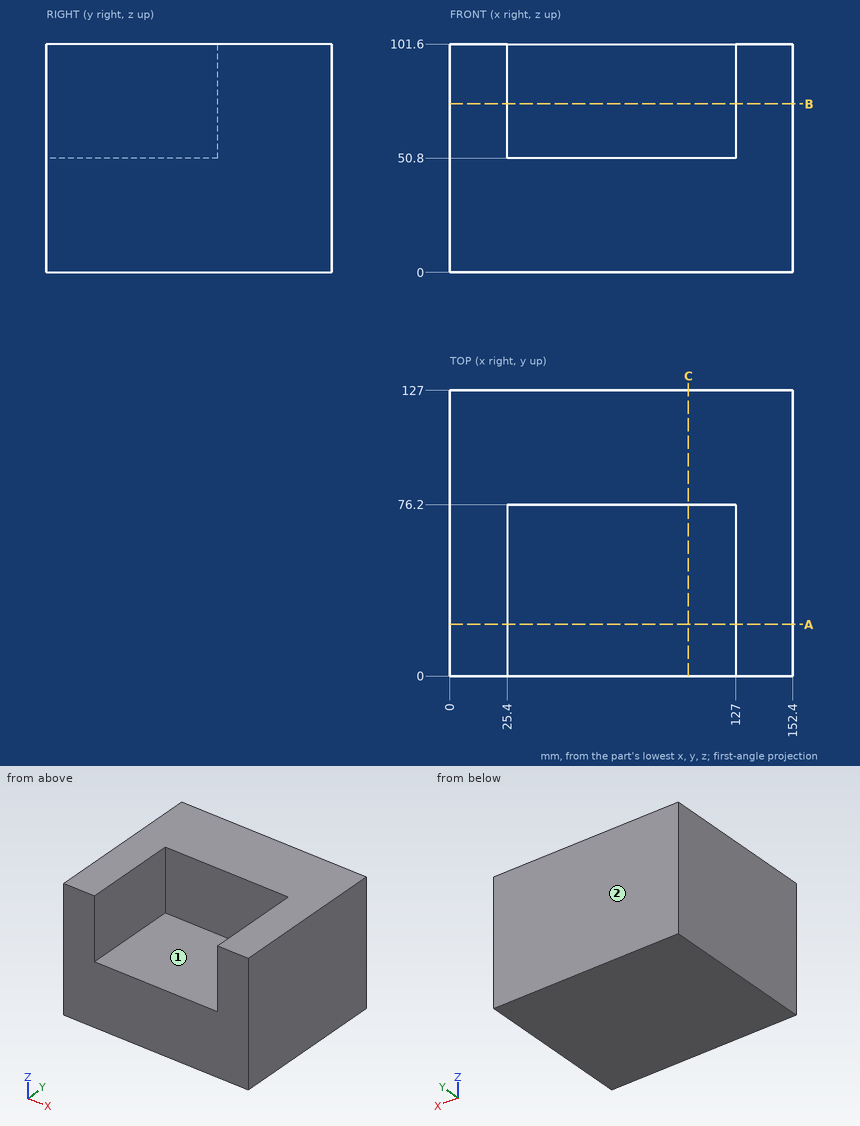
Input: dimensioned drawing with shaded views. Units: mm. Origin: part minimum x, y, z. A direction names the side the tool comes from. Coordinates: 2 decimals unless noted, no trailing zeros. Loops run counter-clockwise (first coordinate to the right, second up) from the corner with the lowest first, then second, coordinate; pieces in that order, holes last.
Q1. Line query: line 1 along X through (y, z) = (34.5, 87.5); line 2 along Y through (x, z) = (110, 74.5); line 3 along Z through (x, y) = (126, 8). Output: solid intervals per line, ascending.
Results are:
line 1: x = 0 to 25.4, 127 to 152.4
line 2: y = 76.2 to 127
line 3: z = 0 to 50.8
Q2. Section C-C, the plane x = 106. Return the cut outline in (y, z).
Results are:
outline: (0, 0) - (127, 0) - (127, 101.6) - (76.2, 101.6) - (76.2, 50.8) - (0, 50.8) - close
Q3. Section A-A, the plane y = 23. Return the cut outline in (x, z), and give its area (3 significant figures).
Results are:
outline: (0, 0) - (152.4, 0) - (152.4, 101.6) - (127, 101.6) - (127, 50.8) - (25.4, 50.8) - (25.4, 101.6) - (0, 101.6) - close
area: 10,300 mm2
Q4. Section B-B, the plane z = 75. Return the cut outline in (x, y), and give its area (3 significant figures).
Results are:
outline: (0, 0) - (25.4, 0) - (25.4, 76.2) - (127, 76.2) - (127, 0) - (152.4, 0) - (152.4, 127) - (0, 127) - close
area: 11,600 mm2
Q5. Set-up query: the marked faces 1 and 2. Return all of +Z, -Z, +X, -X, +Y, -Y with unobstructed straight access to the full face (end or side cutting, diameter ignored); none if empty.
Results are:
face 1: +Z, -Y
face 2: +Z, -Z, +X, -X, +Y
Q6. Contact query for flat-ended pins moving along their axis: pin 1 (5 mm diameter, centred on x = 92, z = 89.5, fed in from -Y); pin 2 (3 mm diameter, centred on x = 65.5, y = 33.5, fed in from +Z). Output: stop coordinate, or through.
Results are:
pin 1: stops at y = 76.2
pin 2: stops at z = 50.8
